Here's how the part is built. I have some questions about the finished solid (model axes, mm). A direction names the side the tool comes from. Round coordinates to 2 decimals unless told otherwise and drop trailing zeros. Loops run counter-clockwise (first coordinate to the right, second up) from the corner with the lowest first, then second, coordinate; pieces in that order, holes last. Notation, with made-up numbers: M -18,-10.75 L 20,-10.75 A23 ccw 20,-2.75 Z; hole C 23.25,-38.75 d9. An arc over 180 degrees is marked long. Answer as a JSON object with one key per item and string values.
from build123d import *

# Parameters (mm, degrees)
F1_DEPTH = 19.05
F2_R     = 2.6543
F3_DEPTH = 54.466987
F4_R     = 4.826
F5_DEPTH = 39.878


with BuildPart() as f1:
    # F0 (on Top) → F1 (new body)
    with BuildSketch(Plane.XY):
        with BuildLine():
            ThreePointArc((-44.250161, 27.048605), (0, 68.814592), (44.250161, 27.048605))
            Line((44.250161, 27.048605), (60.325, 27.048605))
            Line((60.325, 27.048605), (60.325, 52.448605))
            Line((60.325, 52.448605), (49.699983, 52.448605))
            ThreePointArc((49.699983, 52.448605), (0, 81.514592), (-49.699983, 52.448605))
            Line((-49.699983, 52.448605), (-60.325, 52.448605))
            Line((-60.325, 52.448605), (-60.325, 27.048605))
            Line((-60.325, 27.048605), (-44.250161, 27.048605))
        make_face()
    extrude(amount=F1_DEPTH)

    # F2 (on face) → F3 (cut, through all)
    with BuildSketch(Plane.XZ.offset(-27.048605)):
        with Locations((-52.28758, 9.525)):
            Circle(F2_R)
        with Locations((52.287572, 9.525)):
            Circle(F2_R)
    extrude(amount=-F3_DEPTH, mode=Mode.SUBTRACT)

    # F4 (on face) → F5 (cut)
    with BuildSketch(Plane(origin=(0, 52.448605, 0), x_dir=(-1, 0, 0), z_dir=(0, 1, 0))):
        with Locations((-52.287572, 9.525)):
            Circle(F4_R)
        with Locations((52.28758, 9.525)):
            Circle(F4_R)
        with Locations((-52.287572, 79.375)):
            Circle(F4_R)
        with Locations((52.28758, 79.375)):
            Circle(F4_R)
    extrude(amount=F5_DEPTH, mode=Mode.SUBTRACT)


solid = f1.part
Item 1: For P1, Ø6, axis at x = -11, z = 16, coming from the -Y side; P2, Ø3, axis at x = -52.29, z = 9.52, coming from the -Y side; P3, Ø5, axis at x = -16.5, z = 5.5, coming from the -Y side; P4, Ø4, axis at x = 56, z = 13.5, coming from the +Y side, each with a flat end and sliding along its axis, tell me the tip position at first contact or that it passes through.
Solution:
{"P1": "stops at y = 66.55", "P2": "passes through", "P3": "stops at y = 64.54", "P4": "stops at y = 52.45"}
Item 2: I want a section at B-B on y = 61. List the corners of the cut face in (x, z) for me.
Solution:
{"outline": "M -43.8,0 L -25.13,0 L -25.13,19.05 L -43.8,19.05 Z; M 25.13,0 L 43.8,0 L 43.8,19.05 L 25.13,19.05 Z"}
Item 3: For faces 1 (the face through (4, 71, 0)), 2 (the face through (-47.462, 53.843, 9.593)), 3 (the face through (47.462, 53.844, 9.457)), which set-ups out of +Z, -Z, +X, -X, +Y, -Y let a thin tool reach every point of the face, with its end or its side?
Solution:
{"face 1": "-Z, +X, -X, +Y, -Y", "face 2": "-X, +Y", "face 3": "+X, +Y"}
Item 4: I want a section at D-D on x = -52.5. List the corners of the cut face in (y, z) for me, plus the area to 3 significant figures.
Solution:
{"outline": "M 27.05,0 L 52.45,0 L 52.45,6.88 L 27.05,6.88 Z; M 27.05,12.17 L 52.45,12.17 L 52.45,19.05 L 27.05,19.05 Z", "area": "349 mm2"}
Item 5: I want a section at C-C on z = 8. List the corners of the cut face in (x, y) for me (3 decimals).
Solution:
{"outline": "M -60.325,27.049 L -54.46,27.049 L -54.46,52.449 L -60.325,52.449 Z; M -50.115,27.049 L -44.25,27.049 A44.324 cw 44.25,27.049 L 50.115,27.049 L 50.115,52.449 L 47.709,52.449 L 47.709,55.725 A57.024 ccw -47.709,55.725 L -47.709,52.449 L -50.115,52.449 Z; M 54.46,27.049 L 60.325,27.049 L 60.325,52.449 L 54.46,52.449 Z"}
Item 6: I want a section at A-A on y = 48. List the corners of the cut face in (x, z) for me (3 decimals).
Solution:
{"outline": "M -60.325,0 L -37.576,0 L -37.576,19.05 L -60.325,19.05 Z; M 37.576,0 L 60.325,0 L 60.325,19.05 L 37.576,19.05 Z; hole C -52.288,9.525 d5.309; hole C 52.288,9.525 d5.309"}
Item 7: If I drill on L1, parallel to Z at x = -52, y = 38.5; L2, parallel to X at y = 32, z = 2.5 (3 decimals); L3, parallel to X at y = 65, z = 11, over which ranges is the centre line in solid material (lowest first)? Write a range as from..to.
Solution:
{"L1": "z = 0..6.89, 12.16..19.05", "L2": "x = -60.325..-43.683, 43.683..60.325", "L3": "x = -40.13..-17.99, 17.99..40.13"}
Item 8: We'd pull the mould along Y, two halves only. Please class faces 4 (the face through (50, 27.049, 7)), 5 (the face through (55.4, 52.449, 9.4)), 6 (the face through (4, 71, 19.05)): +Y half, -Y half, draft (parallel to the pull), parting line (faces both ways), or undercut.
Solution:
{"face 4": "-Y half", "face 5": "+Y half", "face 6": "draft"}
